```python
from build123d import *

# Parameters (mm, degrees)
F1_DEPTH = 76.2


with BuildPart() as f1:
    # F0 (on Right) → F1 (new body)
    with BuildSketch(Plane.YZ):
        Polygon((-93.878396, 40.8432), (-90.677999, -7.62), (-62.636398, -7.62), (-52.577998, 5.7912), (-21.4884, 5.7912), (-12.0396, -4.8768), (77.571601, -4.8768), (84.582001, 5.7912), (110.794805, 5.7912), (125.425205, -4.8768), (153.162003, -4.8768), (153.162003, 41.148003), (105.708321, 42.520983), (68.884805, 43.586399), (32.613605, 43.586399), (-38.662857, 42.040645), align=None)
        Polygon((0, 61.569601), (-38.662857, 42.040645), (32.613605, 43.586399), (68.884805, 43.586399), (105.708321, 42.520983), (75.590402, 61.569601), align=None)
    extrude(amount=F1_DEPTH)


solid = f1.part
```
Here's how the part is built. I have some questions about the finished solid (model axes, mm). A direction names the side the tool comes from. Coordinates: 2 decimals unless noted, no trailing zeros. Loops run counter-clockwise (first coordinate to the right, second up) from the corner with the lowest first, then second, coordinate; pieces in that order, holes last. Notation, with made-up numbers: M 57,52.25 L 100,52.25 A25 ccw 100,89.25 Z; hole C 79.25,7.25 d10. An arc over 180 degrees is marked long. One line per item, written item: value.
1. On a 3-axis mill with a long thin cutter (end or side, diameter ignored), from which of +Z, -Z, +X, -X, +Y, -Y can I reach the whole of each face in a straight line? I mean faces 4 (the flat face through (38, 139, -4.877)), 5 (the flat face through (38, -37, 5.791)), 6 (the flat face through (76.2, 28, 27)). Say none if no direction works.
Geometry says:
face 4: -Z, +X, -X, +Y
face 5: -Z, +X, -X
face 6: +Z, -Z, +X, +Y, -Y
2. Imagine slicing it at A-A (z = -1). List the corners of the cut face in (x, y) for me.
Geometry says:
outline: M 0,-91.12 L 76.2,-91.12 L 76.2,-57.67 L 0,-57.67 Z; M 0,-15.47 L 76.2,-15.47 L 76.2,80.12 L 0,80.12 Z; M 0,120.11 L 76.2,120.11 L 76.2,153.16 L 0,153.16 Z
3. Will these pins go through, and if not, where does the flat tip stop? pin 1 Ø3 at (x, z) = (39, 9.5) entering from -Y; pin 2 Ø3 at (x, y) = (67, -24.5) entering from -Z; pin 3 Ø23 at (x, y) = (40.5, 17.5) entering from -Z.
Geometry says:
pin 1: stops at y = -91.91
pin 2: stops at z = 5.79
pin 3: stops at z = -4.88
4. Thinking about a two-plate mould opening in Y: for faces 1 (the flat face through (38, -77, -7.62)), 2 (the flat face through (37.57, -19.06, 51.94)), 3 (the flat face through (37.6, -16.8, 0.5)), which applies, +Y half, -Y half, draft (parallel to the pull), parting line (faces both ways), or undercut?
Geometry says:
face 1: draft
face 2: -Y half
face 3: undercut
5. Imagine slicing it at B-B (x = 19.5). List the corners of the cut face in (y, z) for me.
Geometry says:
outline: M -93.88,40.84 L -90.68,-7.62 L -62.64,-7.62 L -52.58,5.79 L -21.49,5.79 L -12.04,-4.88 L 77.57,-4.88 L 84.58,5.79 L 110.79,5.79 L 125.43,-4.88 L 153.16,-4.88 L 153.16,41.15 L 105.71,42.52 L 75.59,61.57 L 0,61.57 L -38.66,42.04 Z
6. Imagine slicing it at C-C (y = 59.5). List the corners of the cut face in (x, z) for me, and give its area (3 significant figures).
Geometry says:
outline: M 0,-4.88 L 76.2,-4.88 L 76.2,61.57 L 0,61.57 Z
area: 5,060 mm2
7. Please list where these lines run through material, in increasing order: probe 1 along Z at (x, y) = (39, 73); probe 2 along Y at (x, z) = (19, -2.5); probe 3 along Z at (x, y) = (31, -82).
Geometry says:
probe 1: z = -4.88 to 61.57
probe 2: y = -91.02 to -58.8, -14.14 to 79.13, 122.17 to 153.16
probe 3: z = -7.62 to 41.1
8. Imagine slicing it at D-D (z = 55). List the corners of the cut face in (x, y) for me.
Geometry says:
outline: M 0,-13.01 L 76.2,-13.01 L 76.2,85.98 L 0,85.98 Z
